Can you work these out from the model? Positions are in its coordinate system, mm. Face numbers are marked on the shaded views. A direction names the side the tool comes from. Round coordinates to 2 decimals unless told otherwise and drop trailing zeros. Loops run counter-clockwise (first coordinate to the right, second up) from the corner with the lowest first, then second, coordinate; pieces in that order, holes last.
from build123d import *

# Parameters (mm, degrees)
S_BOX1_W     = 18
S_BOX1_H     = 2.5
BOSS_1_DEPTH = 80
S_BOX2_W     = 20
S_BOX2_H     = 14.5
BOSS_2_DEPTH = 18
S_HOLE3_R    = 1.5
HOLE_3_DEPTH = 2.7


with BuildPart() as part:
    # S_box1 → Boss_1 (new body)
    with BuildSketch(Plane.XY.offset(-72)):
        with Locations((0, 19.45)):
            Rectangle(S_BOX1_W, S_BOX1_H)
    extrude(amount=BOSS_1_DEPTH)

    # S_box2 → Boss_2 (add)
    with BuildSketch(Plane.XY.offset(-88)):
        with Locations((0, 11.45)):
            Rectangle(S_BOX2_W, S_BOX2_H)
    extrude(amount=BOSS_2_DEPTH)

    # S_hole3 → Hole_3 (cut)
    with BuildSketch(Plane(origin=(0, 18.1, 0), x_dir=(1, 0, 0), z_dir=(0, 1, 0))):
        with Locations(Location((0, 0, 0), (0, 0, 90))):
            Circle(S_HOLE3_R)
    extrude(amount=HOLE_3_DEPTH, mode=Mode.SUBTRACT)


solid = part.part
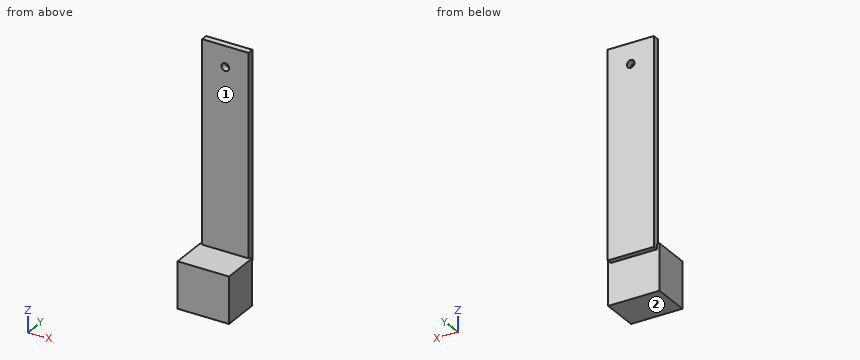
(1) If I drill on line 1 (X direction, y = 19.35, z = 0); line 2 (Y direction, x = 6.5, z = -19); line 3 (Z direction, x = -4.25, y = 9.5), over which ranges is the centre line in solid material (lowest first)?
Worked answers:
line 1: x = -9 to -1.5, 1.5 to 9
line 2: y = 18.2 to 20.7
line 3: z = -88 to -70
(2) If we section it at A-A, the plane x = 0: List the corners of the cut face in (y, z) for me.
Worked answers:
outline: (4.2, -88) - (18.7, -88) - (18.7, -72) - (20.7, -72) - (20.7, -1.5) - (18.2, -1.5) - (18.2, -70) - (4.2, -70) - close; (18.2, 1.5) - (20.7, 1.5) - (20.7, 8) - (18.2, 8) - close
(3) If we section it at C-C, the plane x = 4: List the corners of the cut face in (y, z) for me, then the cut area to 3 significant figures.
Worked answers:
outline: (4.2, -88) - (18.7, -88) - (18.7, -72) - (20.7, -72) - (20.7, 8) - (18.2, 8) - (18.2, -70) - (4.2, -70) - close
area: 460 mm2
(4) If we section it at D-D, the plane y = 6.25: List the corners of the cut face in (x, z) for me, then the cut area to 3 significant figures.
Worked answers:
outline: (-10, -88) - (10, -88) - (10, -70) - (-10, -70) - close
area: 360 mm2
(5) If we section it at B-B, the plane z = 0: List the corners of the cut face in (x, y) for me.
Worked answers:
outline: (-9, 18.2) - (-1.5, 18.2) - (-1.5, 20.7) - (-9, 20.7) - close; (1.5, 18.2) - (9, 18.2) - (9, 20.7) - (1.5, 20.7) - close
(6) For the marked faces 1 and 2, which set-ups out of +Z, -Z, +X, -X, +Y, -Y let a thin tool reach every point of the face, with its end or its side?
Worked answers:
face 1: +Z, +X, -X, -Y
face 2: -Z, +X, -X, +Y, -Y
(7) Will these pins go through, and if not, where does the flat tip stop? P1, Ø5.5, axis at x = 2, z = -41.5, coming from the -Y side; P2, Ø3, axis at y = 20, z = -46, coming from the -X side; P3, Ø1.6, axis at x = -1.5, y = 20, coming from the -Z side; P4, Ø1.8, axis at x = 0, z = 0, coming from the -Y side.
Worked answers:
P1: stops at y = 18.2
P2: stops at x = -9
P3: stops at z = -72
P4: passes through
